Autodesk Inventor part; units mm, degrees
ref_plane "YZ Plane" through (0, 0, 0) normal (1, 0, 0) x (0, 1, 0)
ref_plane "XZ Plane" through (0, 0, 0) normal (0, 1, 0) x (-1, 0, 0)
ref_plane "XY Plane" through (0, 0, 0) normal (0, 0, 1) x (1, 0, 0)
sketch "Sketch1" plane through (0, 0, 0) normal (0, 1, 0) x (-1, 0, 0)
  line L0 (-315.9154, 73.2239) -> (-195.9154, 73.2239)
  line L1 (-195.9154, 73.2239) -> (224.0846, -86.7761)
  line L2 (324.0846, -86.7761) -> (224.0846, -86.7761)
  line L3 (324.0846, -106.7761) -> (220.4041, -106.7761)
  line L4 (220.4041, -106.7761) -> (-199.5959, 53.2239)
  line L5 (-199.5959, 53.2239) -> (-315.9154, 53.2239)
  line L6 (324.0846, -106.7761) -> (324.0846, -86.7761)
  line L7 (-315.9154, 53.2239) -> (-315.9154, 73.2239)
  point P0 (0, 0)
  dimension "d2" = 100
  dimension "d3" = 449.4441
  dimension "d4" = 120
  dimension "d5" = 159.146
  dimension "d6" = 159.146
  dimension "d7" = 20
extrude "Extrusion1" add sketch "Sketch1" along normal blind 70
sketch "Sketch2" plane through (-324.0846, 0, -106.7761) normal (-1, 0, 0) x (0, 0, 1)
  line L0 (0, 48) -> (20, 48)
  line L1 (20, 48) -> (20, 70)
  line L2 (20, 70) -> (0, 70)
  line L3 (0, 70) -> (0, 48)
  point P0 (106.7761, 0)
extrude "Extrusion2" add sketch "Sketch2" along normal blind 110
fillet "Fillet1" radius 30 1 edges at (-324.0846, 48, -96.7761)
properties part number "Y_zigZag" material "Aluminum 6061"
For this review, take the finished solid that the model builds, in its own axes (mm). A direction names the side the tool comes from. Coordinates: 2 decimals unless noted, no trailing zeros. Order: outer loops, then holes, each group sorted by start corner. A loop starts at its lowest first (then second) coordinate and runs counter-clockwise, first axis right, second up. Notation, with made-up numbers: (12, 58.25) -> (50, 58.25) arc R31 ccw to (50, 95.25) -> close; hole circle Ø3 at (26.5, 53.5). An arc over 180 degrees is marked (long way). Return JSON: item names as keys, results as strings.
1. We need section A-A on y = 55. Write out the cut boundary in (x, z).
Answer block:
{"outline": "(-434.08, -106.78) -> (-220.4, -106.78) -> (199.6, 53.22) -> (315.92, 53.22) -> (315.92, 73.22) -> (195.92, 73.22) -> (-224.08, -86.78) -> (-434.08, -86.78) -> close"}
2. For pin 1 Ø6 at (x, z) = (-399.5, -101.5) entering from -Y; pin 2 Ø20 at (y, z) = (8, -95) entering from -X, all flat-tipped, find the tip position at first contact; note any pin that passes through.
Answer block:
{"pin 1": "y = 48", "pin 2": "x = -324.08"}
3. For line 1 (Z direction, x = -250.5, y = 57.5); line 2 (Z direction, x = 257, y = 46), list the stretches that pass through material, from the lowest coordinate up. Write a range as from..to.
Answer block:
{"line 1": "-106.78..-86.78", "line 2": "53.22..73.22"}
4. We need section D-D on z = -9.5. Write out the cut boundary in (x, y), and give its area (3 significant figures).
Answer block:
{"outline": "(-21.23, 0) -> (34.95, 0) -> (34.95, 70) -> (-21.23, 70) -> close", "area": "3,930 mm²"}
5. We need section C-C on y = 9. Write out the cut boundary in (x, z), and give its area (3 significant figures).
Answer block:
{"outline": "(-324.08, -106.78) -> (-220.4, -106.78) -> (199.6, 53.22) -> (315.92, 53.22) -> (315.92, 73.22) -> (195.92, 73.22) -> (-224.08, -86.78) -> (-324.08, -86.78) -> close", "area": "13,400 mm²"}
6. Machinability: for faces 1 (the flat face through (257, 35, 53.224)), 2 (the flat face through (-307, 42, -86.776)), 3 (the flat face through (-394, 48, -97)), 4 (the flat face through (-57, 70, -30)), which of the approach directions +Z, -Z, +X, -X, +Y, -Y give a long, thin tool a straight path to every point of the face, cutting with its end or side? Answer none if there is none.
Answer block:
{"face 1": "-Z, +X, +Y, -Y", "face 2": "+Z, -X, +Y, -Y", "face 3": "+Z, -Z, -X, -Y", "face 4": "+Z, -Z, +X, -X, +Y"}
7. We need section B-B on x = -257. Write out the cut boundary in (y, z), and give its area (3 significant figures).
Answer block:
{"outline": "(0, -106.78) -> (70, -106.78) -> (70, -86.78) -> (0, -86.78) -> close", "area": "1,400 mm²"}
